Geometry: see drawing. Coordinates: mm, zero at the bounding-box minimum. A direction names the side the tool comes from. Coordinates: 2 decimals unless noted, no trailing zeros. Order: outer loops, then holes, each group sorted by start corner. A loop starts at its lowest first (then second) coordinate and runs counter-clockwise, first axis right, second up. Notation, with made-up numbers: (4.25, 35.25) -> (23.25, 35.25) arc R15 cw to (23.25, 61.25) -> close; hole circle Ø2 at (6, 83). An arc over 180 degrees is marked (long way). Use one line per item in the form item = value.
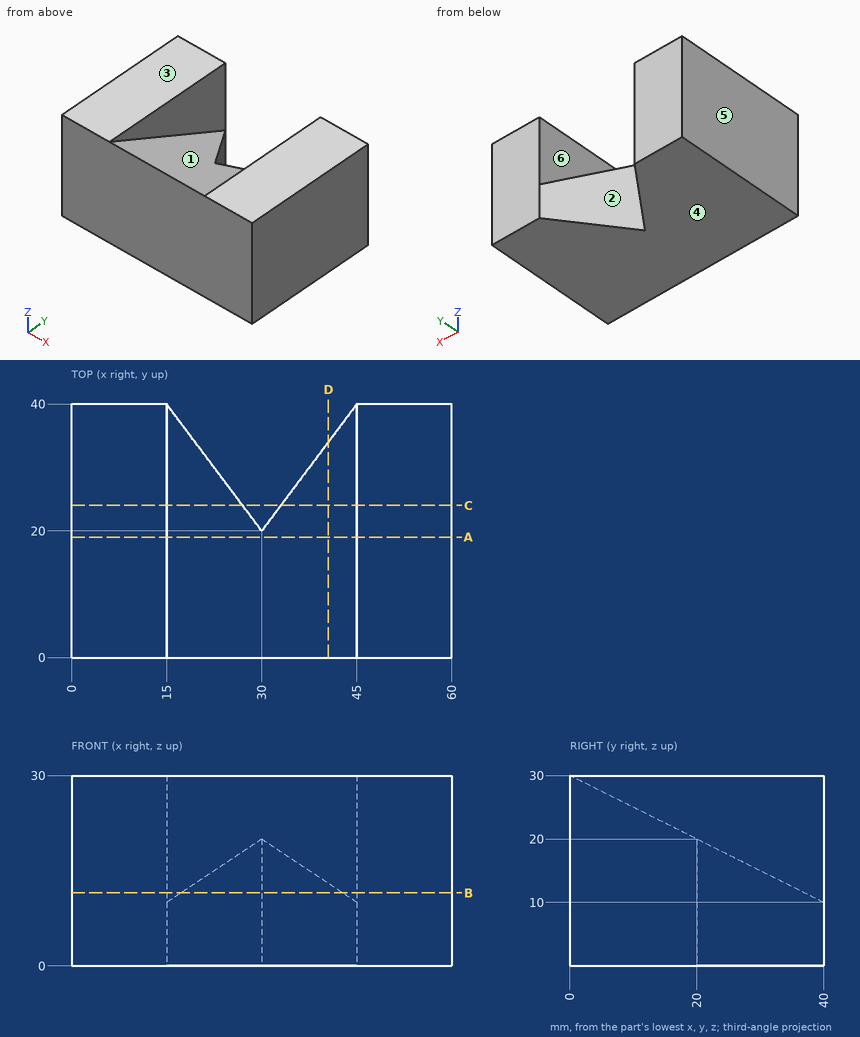
1) Access query for the marked faces 1, 2 and 3. Directions: +Z, -Z, +X, -X, +Y, -Y. A direction counts if a zero-diameter tool reaches every point of the face in a straight line with its end or side. Return the directions, or none.
Results found:
face_1 = +Z, +Y
face_2 = +Z, -Z, +Y
face_3 = +Z, +X, -X, +Y, -Y
2) Material intervals for probe 1 along X at (y, z) = (26, 20.5); probe 2 along Z at (x, y) = (43.5, 30); probe 3 along Z at (x, y) = (16, 7.5), sorted ascending. Write a range as from..to.
Results found:
probe_1 = 0..15, 45..60
probe_2 = 0..15
probe_3 = 0..26.25
3) Section C-C, the plane y = 24. Output: boundary loops of the cut face in (x, z), and give its area (3 significant figures).
Results found:
outline = (0, 0) -> (27, 0) -> (27, 18) -> (15, 18) -> (15, 30) -> (0, 30) -> close; (33, 0) -> (60, 0) -> (60, 30) -> (45, 30) -> (45, 18) -> (33, 18) -> close
area = 1,330 mm2
4) Pull-direction query (X, two-part tool) for the marked faces 4, 5 and 6; classes: released by +X, released by -X, zero draft, split by the parting line, or undercut.
Results found:
face_4 = zero draft
face_5 = released by -X
face_6 = undercut
5) Section B-B, the plane z = 11.5. Output: boundary loops of the cut face in (x, y), and give its area (3 significant figures).
Results found:
outline = (0, 0) -> (60, 0) -> (60, 40) -> (45, 40) -> (45, 37) -> (42.75, 37) -> (30, 20) -> (17.25, 37) -> (15, 37) -> (15, 40) -> (0, 40) -> close
area = 2,090 mm2
6) Section A-A, the plane y = 19. Output: boundary loops of the cut face in (x, z).
Results found:
outline = (0, 0) -> (60, 0) -> (60, 30) -> (45, 30) -> (45, 20.5) -> (15, 20.5) -> (15, 30) -> (0, 30) -> close
7) Section D-D, the plane x = 40.5. Output: boundary loops of the cut face in (y, z).
Results found:
outline = (0, 0) -> (34, 0) -> (34, 13) -> (0, 30) -> close
8) Contact query for a flat-ended pin moving along its axis: P1, Ø12, axis at x = 26.5, z = 6.5, coming from the +Y side. Output: stop coordinate, or through.
Results found:
P1 = 32.67
